from build123d import *

# Parameters (mm, degrees)
SKETCH1_R             = 2.5
BOSS_EXTRUDE1_DEPTH   = 20
M3X0_5_TAPPED_HOLE1_D = 2.5
CHAMFER1_SIZE         = 0.5


with BuildPart() as part:
    # Sketch1 → Boss-Extrude1 (new, symmetric)
    with BuildSketch(Plane.XY):
        Circle(SKETCH1_R)
    extrude(amount=BOSS_EXTRUDE1_DEPTH, both=True)

    # M3x0.5 Tapped Hole1 (through all)
    with Locations(Plane.XY.offset(20)):
        with Locations((0, 0)):
            Hole(M3X0_5_TAPPED_HOLE1_D / 2)

    # Chamfer1
    chamfer1_edges = [part.edges().sort_by_distance(p)[0] for p in [
        (-2.5, 0, -20),
        (-2.5, 0, 20),
    ]]
    chamfer(chamfer1_edges, length=CHAMFER1_SIZE)


solid = part.part
The model under review builds one solid part; all positions refer to its coordinate system, in mm. Give positions to 0.01 mm unless a question says otherwise; leave off trailing zeros. Write each loop counter-clockwise with the first axis right and the second up, starting at its lowest first coordinate (ties: lowest second). Pieces come first, ordered by that corner, then holes.
1. For P1, Ø1.5, axis at x = -1.5, z = 13.5, coming from the -Y side; P2, Ø1.5, axis at x = -1.5, z = 0.5, coming from the +Y side; P3, Ø3, axis at x = 0, y = 0, coming from the -Z side, all flat-tipped, find the tip position at first contact; note any pin that passes through.
2. Add section C-C, the plane z = -13. Write out the cut boundary in (x, y), plus the area to 3 significant figures.
3. Draft analysis for pull direction Y (two halves, no side actions). For faces 1 (the flat face through (1, 1, -20)), 2 (the cylindrical face through (0.27, -1.22, -0.28)), 3 (the cylindrical face through (-0.54, -2.44, 0.27)), state which applies: +Y half, -Y half, draft (parallel to the pull), parting line (faces both ways), or undercut.
4. Wall thickness on L1, parallel to Y at x = 0, z = 3; L2, parallel to X at y = 0.9, z = 6.5: over which ranges is each line inside the solid? List them lowest first.
5. Add section A-A, the plane y = 0. Write out the cut boundary in (x, z).
Worked answers:
1. P1: stops at y = -2.38
1. P2: stops at y = 2.38
1. P3: stops at z = -20
2. outline: circle Ø5 at (0, 0); hole circle Ø2.5 at (0, 0)
2. area: 14.7 mm2
3. face 1: draft
3. face 2: undercut
3. face 3: parting line
4. L1: y = -2.5 to -1.25, 1.25 to 2.5
4. L2: x = -2.33 to -0.87, 0.87 to 2.33
5. outline: (-2.5, -19.5) - (-2, -20) - (-1.25, -20) - (-1.25, 20) - (-2, 20) - (-2.5, 19.5) - close; (1.25, -20) - (2, -20) - (2.5, -19.5) - (2.5, 19.5) - (2, 20) - (1.25, 20) - close
